from build123d import *

# Parameters (mm, degrees)
SKETCH1_R           = 45
SKETCH1_R_2         = 5
BOSS_EXTRUDE1_DEPTH = 15
SKETCH3_R           = 25
BOSS_EXTRUDE2_DEPTH = 35
FILLET1_R           = 1
CHAMFER1_SIZE       = 1
SKETCH4_R           = 17.5
CUT_EXTRUDE1_DEPTH  = 59


with BuildPart() as part:
    # Sketch1 → Boss-Extrude1 (new body)
    with BuildSketch(Plane.XY):
        Circle(SKETCH1_R)
        with Locations((0, 32.5)):
            Circle(SKETCH1_R_2, mode=Mode.SUBTRACT)
        with Locations((32.5, 0)):
            Circle(SKETCH1_R_2, mode=Mode.SUBTRACT)
        with Locations((0, -32.5)):
            Circle(SKETCH1_R_2, mode=Mode.SUBTRACT)
        with Locations((-32.5, 0)):
            Circle(SKETCH1_R_2, mode=Mode.SUBTRACT)
    extrude(amount=-BOSS_EXTRUDE1_DEPTH)

    # Sketch3 → Boss-Extrude2 (add)
    with BuildSketch(Plane(origin=(0, 0, -15), x_dir=(-1, 0, 0), z_dir=(0, 0, -1))):
        with Locations(Location((0, 0, 0), (0, 0, 180))):
            Circle(SKETCH3_R)
    extrude(amount=BOSS_EXTRUDE2_DEPTH)

    # Fillet1
    fillet1_edges = [part.edges().sort_by_distance(p)[0] for p in [
        (-25, 0, -15),
    ]]
    fillet(fillet1_edges, radius=FILLET1_R)

    # Chamfer1
    chamfer1_edges = [part.edges().sort_by_distance(p)[0] for p in [
        (-45, 0, -15),
    ]]
    chamfer(chamfer1_edges, length=CHAMFER1_SIZE)

    # Sketch4 → Cut-Extrude1 (cut)
    with BuildSketch(Plane(origin=(0, 0, -50), x_dir=(-1, 0, 0), z_dir=(0, 0, -1))):
        Circle(SKETCH4_R)
    extrude(amount=-CUT_EXTRUDE1_DEPTH, mode=Mode.SUBTRACT)


solid = part.part
Model file for the job. Use its own axes, mm. Round coordinates to 2 decimals unless told otherwise and drop trailing zeros. Loops run counter-clockwise (first coordinate to the right, second up) from the corner with the lowest first, then second, coordinate; pieces in that order, holes last. Notation, with made-up numbers: M -1,0.5 L 38,0.5 A11 cw 38,21.5 Z; hole C 47,-26.5 d5. An arc over 180 degrees is marked long. One line per question, with ' | ' between items.
1) Flat gauge pins, fed straight in: pin 1 (12 mm diameter, centred on x = -34, z = -19.5, fed in from +Y); pin 2 (13 mm diameter, centred on x = -32.5, y = 0, fed in from -Z); pin 3 (1.5 mm diameter, centred on x = -5.5, z = -20.5, fed in from +Y). Where does each tip first touch, or does it go through?
Solved:
pin 1: stops at y = 32.23 | pin 2: stops at z = -15 | pin 3: stops at y = 24.54
2) Band-saw the part on A-A (y = 0). Give the cut face in (x, z).
Solved:
outline: M -45,-14 L -44,-15 L -37.5,-15 L -37.5,0 L -45,0 Z; M -27.5,-15 L -26,-15 A1 cw -25,-16 L -25,-50 L -17.5,-50 L -17.5,0 L -27.5,0 Z; M 17.5,-50 L 25,-50 L 25,-16 A1 cw 26,-15 L 27.5,-15 L 27.5,0 L 17.5,0 Z; M 37.5,-15 L 44,-15 L 45,-14 L 45,0 L 37.5,0 Z
3) Band-saw the part on C-C (z = -40). Give the cut face in (x, y).
Solved:
outline: C 0,0 d50; hole C 0,0 d35
4) Drill centre lines: line 1 along X through (y, z) = (0.5, -11.5); line 2 along Z through (x, y) = (0, 41.5); line 3 along X through (y, z) = (-4, -38.5). Where is each one in solid material? Low to high.
Solved:
line 1: x = -45 to -37.47, -27.53 to -17.49, 17.49 to 27.53, 37.47 to 45 | line 2: z = -15 to 0 | line 3: x = -24.68 to -17.04, 17.04 to 24.68
5) Mould opens along Y. For faces 1 (the cylindrical face through (-37.495, 0.22, -7.395)), 2 (the flat face through (19, -19, -15)), 3 (the cylindrical face through (23.846, -7.509, -32.762)) say: +Y half, -Y half, draft (parallel to the pull), parting line (faces both ways), or undercut.
Solved:
face 1: undercut | face 2: draft | face 3: parting line
